from build123d import *

# Parameters (mm, degrees)
F0_W     = 75.315695256
F0_H     = 72.1342116594
F1_DEPTH = 254
F2_SIZE  = 12.7
F3_W     = 48.0028837919
F3_H     = 27.0442329347
F4_DEPTH = 25
F5_T     = -2.5
F6_R     = 5
F7_W     = 29.8640429974
F7_H     = 26.566028595
F8_DEPTH = 25


with BuildPart() as f1:
    # F0 (on Right) → F1 (new body)
    with BuildSketch(Plane.YZ):
        with Locations((98.0980489403, 22.5397534668)):
            Rectangle(F0_W, F0_H)
    extrude(amount=F1_DEPTH)

    # F2
    f2_edges = [f1.edges().sort_by_distance(p)[0] for p in [
        (127, 135.755897, 58.606859),
    ]]
    chamfer(f2_edges, length=F2_SIZE)

    # F3 (on face) → F4 (cut)
    with BuildSketch(Plane.XZ.offset(-60.4402013123)):
        with Locations((115.4388412833, 23.4042126685)):
            Rectangle(F3_W, F3_H)
    extrude(amount=-F4_DEPTH, mode=Mode.SUBTRACT)

    # F5
    f5_openings = [f1.faces().sort_by_distance(p)[0] for p in [
        (254, 97.59442, 22.060093),
    ]]
    offset(amount=F5_T, openings=f5_openings, kind=Kind.INTERSECTION)

    # F6
    f6_edges = [f1.edges().sort_by_distance(p)[0] for p in [
        (127, 60.440201, -13.527352),
        (127, 60.440201, 58.606859),
        (127, 135.755897, -13.527352),
    ]]
    fillet(f6_edges, radius=F6_R)

    # F7 (on face) → F8 (cut)
    with BuildSketch(Plane.XZ.offset(-60.4402013123)):
        with Locations((205.0164192915, 28.6153107882)):
            Rectangle(F7_W, F7_H)
    extrude(amount=-F8_DEPTH, mode=Mode.SUBTRACT)


solid = f1.part
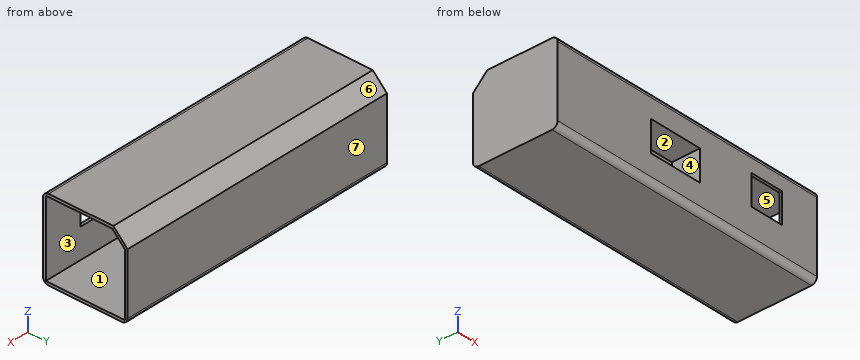
Can you work these out from the model? Positions are in its coordinate system, mm. Face numbers are marked on the shaded views. A direction names the side the tool comes from. Coordinates: 2 decimals unless noted, no trailing zeros. Loops run counter-clockwise (first coordinate to the right, second up) from the corner with the lowest first, then second, coordinate; pieces in that order, holes last. Notation, with made-up numbers: (-4, -24) - (43, -24) arc R18 cw to (43, -2) - close; hole circle Ø11 at (31, 19). An arc over 180 degrees is marked (long way). Answer as a JSON object with one key per item and string values. Group by question number.
Item 1: If we section it at C-C (x = 118): List the corners of the cut face in (y, z) for me.
Item 2: If we section it at A-A (z = 33.5): List the corners of the cut face in (x, y) for me, plus the area to 3 significant figures.
Item 3: If we section it at D-D (x = 216): List the corners of the cut face in (y, z) for me.
Item 4: If we mould it in two halves opening along Z, with no side actions, what happens to the marked faces 4, 5, 6 and 7? For each: released by +Z, released by -Z, zero draft, split by the parting line, or undercut.
Item 5: On a 3-axis mill with a long thin cutter (end or side, diameter ignored), from which of +Z, -Z, +X, -X, +Y, -Y can I reach the whole of each face in a straight line? I mean the marked faces 1, 2 and 3. Say none if no direction works.
Item 6: If we section it at B-B (y = 82.5): List the corners of the cut face in (x, z) for me.
Item 7: For pin 1 (3 mm diameter, centred on y = 77, z = 32.5, fed in from +X); pin 2 (13.5 mm diameter, centred on x = 104.5, z = 24.5, fed in from -Y); pin 3 (1 mm diameter, centred on y = 118, z = -0.5, fed in from +X), each with a flat end and sliding along its axis, tell me the tip position at first contact or that it passes through.
Item 8: If I drill on L1, parallel to X at y = 71, z = 25; L2, parallel to Y at x = 106, z = -3; L3, parallel to Z at x = 89, y = 115.5, over which ranges is the centre line in solid material (lowest first)? Write a range as from..to.
Returned:
{
 "1": {"outline": "(60.44, -8.53) arc R5 ccw to (65.44, -13.53) - (130.76, -13.53) arc R5 ccw to (135.76, -8.53) - (135.76, 45.91) - (123.06, 58.61) - (65.44, 58.61) arc R5 ccw to (60.44, 53.61) - (60.44, 36.93) - (85.44, 36.93) - (85.44, 9.88) - (60.44, 9.88) - close; hole (62.94, -11.03) - (133.26, -11.03) - (133.26, 44.87) - (122.02, 56.11) - (62.94, 56.11) - (62.94, 39.43) - (87.94, 39.43) - (87.94, 7.38) - (62.94, 7.38) - close"},
 "2": {"outline": "(0, 60.44) - (91.44, 60.44) - (91.44, 85.44) - (139.44, 85.44) - (139.44, 60.44) - (190.08, 60.44) - (190.08, 62.94) - (141.94, 62.94) - (141.94, 87.94) - (88.94, 87.94) - (88.94, 62.94) - (2.5, 62.94) - (2.5, 133.26) - (254, 133.26) - (254, 135.76) - (0, 135.76) - close; (219.95, 60.44) - (254, 60.44) - (254, 62.94) - (219.95, 62.94) - close", "area": "1,500 mm²"},
 "3": {"outline": "(60.44, -8.53) arc R5 ccw to (65.44, -13.53) - (130.76, -13.53) arc R5 ccw to (135.76, -8.53) - (135.76, 45.91) - (123.06, 58.61) - (65.44, 58.61) arc R5 ccw to (60.44, 53.61) - (60.44, 41.9) - (62.94, 41.9) - (62.94, 56.11) - (122.02, 56.11) - (133.26, 44.87) - (133.26, -11.03) - (62.94, -11.03) - (62.94, 15.33) - (60.44, 15.33) - close"},
 "4": {"face 4": "undercut", "face 5": "undercut", "face 6": "released by +Z", "face 7": "zero draft"},
 "5": {"face 1": "+X", "face 2": "-Y", "face 3": "none"},
 "6": {"outline": "(0, -13.53) - (254, -13.53) - (254, -11.03) - (2.5, -11.03) - (2.5, 56.11) - (254, 56.11) - (254, 58.61) - (0, 58.61) - close; (88.94, 7.38) - (141.94, 7.38) - (141.94, 39.43) - (88.94, 39.43) - close; hole (91.44, 9.88) - (139.44, 9.88) - (139.44, 36.93) - (91.44, 36.93) - close"},
 "7": {"pin 1": "stops at x = 141.94", "pin 2": "stops at y = 85.44", "pin 3": "stops at x = 2.5"},
 "8": {"L1": "x = 0..2.5, 88.94..91.44, 139.44..141.94", "L2": "y = 60.44..62.94, 133.26..135.76", "L3": "z = -13.53..-11.03, 56.11..58.61"}
}
